Could you check a few things on this model? Use its own coordinates, in mm. Coordinates: 2 decimals unless noted, no trailing zeros. Order: outer loops, then holes, each group sorted by start corner. A loop starts at its lowest first (then second) coordinate and runs counter-clockwise, first axis right, second up. Notation, with made-up numbers: (39, 45.25) -> (51, 45.25) arc R25 cw to (51, 57.25) -> close; hole circle Ø7 at (57, 27). An arc over 180 degrees is marked (long way). Put each result on its own line as item: value. Start each with the question number.
Q1. Will these pins go through, and if not, where does the flat tip stop? pin 1 (4 mm diameter, centred on y = 6, z = 103.5, fed in from -X) (3 decimals); pin 2 (3 mm diameter, centred on x = 14.5, y = 23, fed in from +Z).
Q2. If we section it at B-B (x = 21.5): Please give me the cut outline in (y, z) (3 decimals), and give its area (3 significant figures).
Q3. If we section it at A-A (z = 57.15): Please give me the cut outline in (x, y) (3 decimals).
Q4. Please list where these lines run through material, in increasing order: line 1 along X through (y, z) = (1.6, 69.85); line 2 along Y through (x, z) = (39.5, 110) (3 decimals); line 3 along X through (y, z) = (8.5, 20) (3 decimals).
Q5. If we section it at C-C (y = 10.5): Please give me the cut outline in (x, z) (3 decimals).
Q6. If we section it at D-D (x = 38.1): Please give me the cut outline in (y, z) (3 decimals), and give its area (3 significant figures).
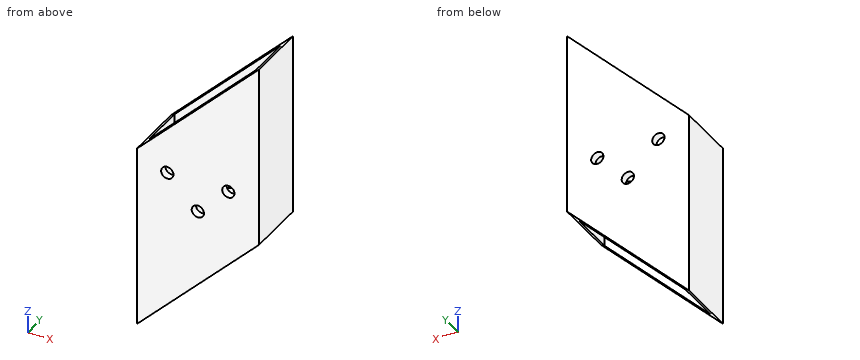
from build123d import *

# Parameters (mm, degrees)
SKETCH1_W           = 50.8
SKETCH1_H           = 25.4
SKETCH1_W_2         = 44.45
SKETCH1_H_2         = 19.05
BOSS_EXTRUDE1_DEPTH = 127
CUT_EXTRUDE1_DEPTH  = 127
SKETCH3_R           = 2.5527
CUT_EXTRUDE2_DEPTH  = 25.4


with BuildPart() as part:
    # Sketch1 → Boss-Extrude1 (new body)
    with BuildSketch(Plane.XY):
        with Locations((25.4, 12.7)):
            Rectangle(SKETCH1_W, SKETCH1_H)
        with Locations((25.4, 12.7)):
            Rectangle(SKETCH1_W_2, SKETCH1_H_2, mode=Mode.SUBTRACT)
    extrude(amount=BOSS_EXTRUDE1_DEPTH)

    # Sketch2 → Cut-Extrude1 (cut)
    with BuildSketch(Plane(origin=(0, 25.4, 0), x_dir=(1, 0, 0), z_dir=(0, 1, 0))):
        Polygon((0, 0), (50.8, -50.8), (50.8, 0), align=None)
        Polygon((0, -76.2), (0, -127), (50.8, -127), align=None)
    extrude(amount=-CUT_EXTRUDE1_DEPTH, mode=Mode.SUBTRACT)

    # Sketch3 → Cut-Extrude2 (cut)
    with BuildSketch(Plane(origin=(0, 25.4, 0), x_dir=(1, 0, 0), z_dir=(0, 1, 0))):
        with Locations((12.7, -69.85)):
            Circle(SKETCH3_R)
        with Locations((38.1, -69.85)):
            Circle(SKETCH3_R)
        with Locations((25.4, -57.15)):
            Circle(SKETCH3_R)
    extrude(amount=-CUT_EXTRUDE2_DEPTH, mode=Mode.SUBTRACT)


solid = part.part
The answers:
1. pin 1: x = 47.625
1. pin 2: z = 92.2
2. outline: (0, 21.5) -> (3.175, 21.5) -> (3.175, 97.7) -> (0, 97.7) -> close; (22.225, 21.5) -> (25.4, 21.5) -> (25.4, 97.7) -> (22.225, 97.7) -> close
2. area: 484 mm^2
3. outline: (0, 0) -> (22.847, 0) -> (22.847, 3.175) -> (3.175, 3.175) -> (3.175, 22.225) -> (22.847, 22.225) -> (22.847, 25.4) -> (0, 25.4) -> close; (27.953, 0) -> (50.8, 0) -> (50.8, 25.4) -> (27.953, 25.4) -> (27.953, 22.225) -> (47.625, 22.225) -> (47.625, 3.175) -> (27.953, 3.175) -> close
4. line 1: 0 to 10.15, 15.25 to 35.55, 40.65 to 50.8
4. line 2: 0 to 3.175, 22.225 to 25.4
4. line 3: 0 to 3.175
5. outline: (0, 0) -> (3.175, 3.175) -> (3.175, 79.375) -> (0, 76.2) -> close; (47.625, 47.625) -> (50.8, 50.8) -> (50.8, 127) -> (47.625, 123.825) -> close
6. outline: (0, 38.1) -> (3.175, 38.1) -> (3.175, 67.297) -> (0, 67.297) -> close; (0, 72.403) -> (3.175, 72.403) -> (3.175, 114.3) -> (0, 114.3) -> close; (22.225, 38.1) -> (25.4, 38.1) -> (25.4, 67.297) -> (22.225, 67.297) -> close; (22.225, 72.403) -> (25.4, 72.403) -> (25.4, 114.3) -> (22.225, 114.3) -> close
6. area: 451 mm^2
